Design review of the part built by this model. Coordinates are the model's own, in mm. A direction names the side the tool comes from. Coordinates: 2 decimals unless noted, no trailing zeros. Write each loop counter-clockwise with the first axis right and the second up, starting at its lowest first coordinate (ties: lowest second). Pieces come first, ordered by that corner, then holes. Notation, with made-up numbers: M 62.25,-1 L 105.25,-1 A19 ccw 105.25,12 Z; hole C 28.5,66 d7. An arc over 180 degrees is marked long. Write item = value, one per line.
```python
from build123d import *

# Parameters (mm, degrees)
CROQUIS1_W              = 50.8
CROQUIS1_H              = 80
SALIENTE_EXTRUIR1_DEPTH = 6.35
CROQUIS4_R              = 4
CORTAR_EXTRUIR3_DEPTH   = 48.806720239
CROQUIS5_W              = 50.8
CROQUIS5_H              = 12.7
CORTAR_EXTRUIR4_DEPTH   = 48.806720239
CROQUIS6_W              = 50.8
CROQUIS6_H              = 20.526572449
CORTAR_EXTRUIR5_DEPTH   = 10
CROQUIS7_W              = 50.8
CROQUIS7_H              = 6.773427551
CORTAR_EXTRUIR6_DEPTH   = 10
CROQUIS8_R              = 3.175
SALIENTE_EXTRUIR2_DEPTH = 10
CROQUIS9_R              = 7
CORTAR_EXTRUIR7_DEPTH   = 10
CROQUIS10_R             = 2
CORTAR_EXTRUIR8_DEPTH   = 10


with BuildPart() as part:
    # Croquis1 → Saliente-Extruir1 (new body)
    with BuildSketch(Plane(origin=(0, 0, 0), x_dir=(1, 0, 0), z_dir=(0, 1, 0))):
        Rectangle(CROQUIS1_W, CROQUIS1_H)
    extrude(amount=SALIENTE_EXTRUIR1_DEPTH)

    # Croquis4 → Cortar-Extruir3 (cut, through all)
    with BuildSketch(Plane(origin=(0, 6.35, 0), x_dir=(1, 0, 0), z_dir=(0, 1, 0))):
        with Locations(Location((-19, 19.466091849, 0), (0, 0, 270))):
            Circle(CROQUIS4_R)
        with Locations(Location((19, 19.466091849, 0), (0, 0, 270))):
            Circle(CROQUIS4_R)
        with Locations(Location((0, 0.466091849, 0), (0, 0, 270))):
            Circle(CROQUIS4_R)
    extrude(amount=-CORTAR_EXTRUIR3_DEPTH, mode=Mode.SUBTRACT)

    # Croquis5 → Cortar-Extruir4 (cut, through all)
    with BuildSketch(Plane(origin=(0, 6.35, 0), x_dir=(1, 0, 0), z_dir=(0, 1, 0))):
        with Locations((0, -33.65)):
            Rectangle(CROQUIS5_W, CROQUIS5_H)
    extrude(amount=-CORTAR_EXTRUIR4_DEPTH, mode=Mode.SUBTRACT)

    # Croquis6 → Cortar-Extruir5 (cut)
    with BuildSketch(Plane(origin=(0, 6.35, 0), x_dir=(1, 0, 0), z_dir=(0, 1, 0))):
        with Locations((0, -17.036713776)):
            Rectangle(CROQUIS6_W, CROQUIS6_H)
    extrude(amount=-CORTAR_EXTRUIR5_DEPTH, mode=Mode.SUBTRACT)

    # Croquis7 → Cortar-Extruir6 (cut)
    with BuildSketch(Plane.XZ):
        with Locations((0, -36.613286225)):
            Rectangle(CROQUIS7_W, CROQUIS7_H)
    extrude(amount=-CORTAR_EXTRUIR6_DEPTH, mode=Mode.SUBTRACT)

    # Croquis8 → Saliente-Extruir2 (add)
    with BuildSketch(Plane(origin=(0, 0, -33.226572449), x_dir=(-1, 0, 0), z_dir=(0, 0, -1))):
        with Locations(Location((0, 3.175, 0), (0, 0, 270))):
            Circle(CROQUIS8_R)
    extrude(amount=SALIENTE_EXTRUIR2_DEPTH)

    # Croquis9 → Cortar-Extruir7 (cut)
    with BuildSketch(Plane.XZ):
        with Locations(Location((0, -19.466091849, 0), (0, 0, 270))):
            Circle(CROQUIS9_R)
    extrude(amount=-CORTAR_EXTRUIR7_DEPTH, mode=Mode.SUBTRACT)

    # Croquis10 → Cortar-Extruir8 (cut)
    with BuildSketch(Plane.XZ):
        with Locations(Location((-20.4, 1.773427551, 0), (0, 0, 270))):
            Circle(CROQUIS10_R)
        with Locations(Location((19.6, 1.773427551, 0), (0, 0, 270))):
            Circle(CROQUIS10_R)
        with Locations(Location((19.6, -28.226572449, 0), (0, 0, 270))):
            Circle(CROQUIS10_R)
        with Locations(Location((-20.4, -28.226572449, 0), (0, 0, 270))):
            Circle(CROQUIS10_R)
    extrude(amount=-CORTAR_EXTRUIR8_DEPTH, mode=Mode.SUBTRACT)


solid = part.part
```
Q1. Wall thickness on line 1 (Z direction, x = 20.5, y = 2); line 2 (X direction, y = 4.75, z = -27.5); line 3 (X direction, y = 4, z = -23): over which ranges is each line inside the solid? List them lowest first.
Check result:
line_1 = -33.23 to -30.01, -26.44 to -23.17, -15.76 to -0.01, 3.56 to 6.77
line_2 = -25.4 to -22.26, -18.54 to 17.74, 21.46 to 25.4
line_3 = -25.4 to -20.87, -17.13 to -6.04, 6.04 to 17.13, 20.87 to 25.4
Q2. Consider section C-C, the plane y = 3. State how many separate pieces and enclosed holes the cut face has, and give its area (3 significant figures).
Check result:
separate_pieces = 1
enclosed_holes = 8
area = 1,740 mm²
Q3. Consider section A-A, the plane z = -14. State the section outline as (x, y) points.
Check result:
outline = M -25.4,0 L -4.37,0 L -4.37,6.35 L -25.4,6.35 Z; M 4.37,0 L 25.4,0 L 25.4,6.35 L 4.37,6.35 Z
Q4. For P1, Ø1.9, axis at x = 9, y = 3.5, coming from the -Z side, flat-tipped, find the tip position at first contact; note if it passes through.
Check result:
P1 = -33.23
Q5. Consider section B-B, the plane x = 19. State the section outline as (y, z) points.
Check result:
outline = M 0,-33.23 L 6.35,-33.23 L 6.35,-30.13 L 0,-30.13 Z; M 0,-26.32 L 6.35,-26.32 L 6.35,-23.47 L 0,-23.47 Z; M 0,-15.47 L 6.35,-15.47 L 6.35,-0.13 L 0,-0.13 Z; M 0,3.68 L 6.35,3.68 L 6.35,6.77 L 0,6.77 Z
Q6. The part is to be moulded in two halves that separate along Z. For faces 3 (the cylindrical face through (-3.905, 3.219, -1.333)), 4 (the flat face through (0, 3, 6.773)), 5 (the flat face through (0, 6.35, -9)), say which applies: +Z half, -Z half, draft (parallel to the pull), parting line (faces both ways), or undercut.
Check result:
face_3 = undercut
face_4 = +Z half
face_5 = draft
Q7. Machinability: for faces 1 (the cylindrical face through (-22.2, 3.1, 0.9)), 2 (the cylindrical face through (-0.954, 0.147, -38.157)), which of the approach directions +Z, -Z, +X, -X, +Y, -Y give a long, thin tool a straight path to every point of the face, cutting with its end or side? Answer none if there is none.
Check result:
face_1 = +Y, -Y
face_2 = -Z
Q8. Consider section D-D, the plane z = 2. State the section outline as (x, y) points.
Check result:
outline = M -25.4,0 L -22.39,0 L -22.39,6.35 L -25.4,6.35 Z; M -18.41,0 L -3.15,0 L -3.15,6.35 L -18.41,6.35 Z; M 3.15,0 L 17.61,0 L 17.61,6.35 L 3.15,6.35 Z; M 21.59,0 L 25.4,0 L 25.4,6.35 L 21.59,6.35 Z
